Here's how the part is built. I have some questions about the finished solid (model axes, mm). Face numbers are marked on the shaded views. A direction names the side the tool comes from. Round coordinates to 2 decimals unless told otherwise and drop trailing zeros. Loops run counter-clockwise (first coordinate to the right, second up) from the corner with the lowest first, then second, coordinate; pieces in that order, holes last. Notation, with made-up numbers: M -10,-26.5 L 15,-26.5 A17 ccw 15,-13.5 Z; hole C 6,3 d1. An arc over 180 degrees is marked long. Use a Markdown table: item, result.
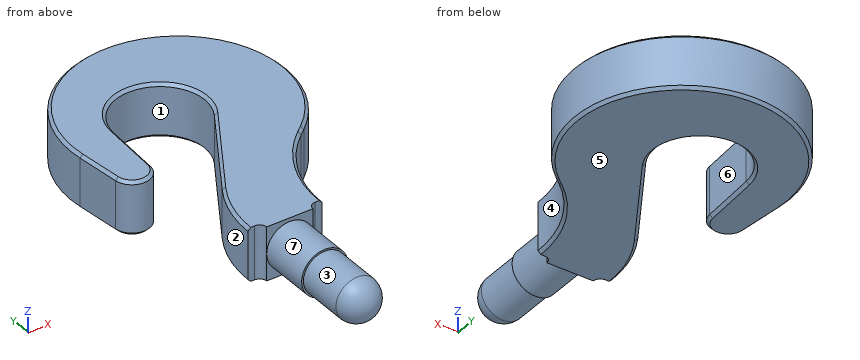
from build123d import *

# Parameters (mm, degrees)
BOSS_EXTRUDE1_DEPTH = 15
CHAMFER1_SIZE       = 0.8
SKETCH2_R           = 6.5
BOSS_EXTRUDE2_DEPTH = 14
SKETCH3_R           = 6
BOSS_EXTRUDE3_DEPTH = 13
DOME1_FACE_RADIUS   = 6
DOME1_HEIGHT        = 5.61


with BuildPart() as part:
    # Sketch1 → Boss-Extrude1 (new body)
    with BuildSketch(Plane.XY):
        with BuildLine():
            Line((5.33, -50.05), (3.429374902, -50.05))
            ThreePointArc((3.429374902, -50.05), (2.032950898, -50.618217894), (1.43, -52))
            Line((1.43, -52), (-11.57, -52))
            ThreePointArc((-11.57, -52), (-12.172950898, -50.618217894), (-13.569374902, -50.05))
            Line((-13.569374902, -50.05), (-15.47, -50.05))
            ThreePointArc((-15.47, -50.05), (-14.21947106, -41.051606397), (-10.562661368, -32.73519774))
            Line((-10.562661368, -32.73519774), (5.571159609, -6.55863722))
            ThreePointArc((5.571159609, -6.55863722), (-1.303288682, 11.918971677), (-17.547628929, 0.747513411))
            Line((-17.547628929, 0.747513411), (-18.508948428, -15.299005365))
            ThreePointArc((-18.508948428, -15.299005365), (-23.375545829, -19.998450876), (-28.469986749, -15.547020759))
            Line((-28.469986749, -15.547020759), (-29.819920496, -3.282124556))
            ThreePointArc((-29.819920496, -3.282124556), (11.287126383, 27.795697113), (19.089371058, -23.142945202))
            Line((19.089371058, -23.142945202), (17.331691836, -24.592760278))
            ThreePointArc((17.331691836, -24.592760278), (8.480844489, -35.977760828), (5.33, -50.05))
        make_face()
    extrude(amount=BOSS_EXTRUDE1_DEPTH)

    # Chamfer1
    chamfer1_edges = [part.edges().sort_by_distance(p)[0] for p in [
        (11.287126383, 27.795697113, 15),
        (-29.144953623, -9.414572658, 15),
        (-14.21947106, -41.051606397, 0),
        (-2.495750879, -19.64691748, 0),
        (-1.303288682, 11.918971677, 0),
        (-18.028288679, -7.275745977, 0),
        (-23.375545829, -19.998450876, 15),
        (-23.375545829, -19.998450876, 0),
        (-29.144953623, -9.414572658, 0),
        (11.287126383, 27.795697113, 0),
        (18.210531447, -23.86785274, 0),
        (8.480844489, -35.977760828, 0),
        (-18.028288679, -7.275745977, 15),
        (-1.303288682, 11.918971677, 15),
        (-2.495750879, -19.64691748, 15),
        (-14.21947106, -41.051606397, 15),
        (8.480844489, -35.977760828, 15),
        (18.210531447, -23.86785274, 15),
    ]]
    chamfer(chamfer1_edges, length=CHAMFER1_SIZE)

    # Sketch2 → Boss-Extrude2 (add)
    with BuildSketch(Plane.XZ.offset(52)):
        with Locations(Location((-5.07, 7.5, 0), (0, 0, 180))):
            Circle(SKETCH2_R)
    extrude(amount=BOSS_EXTRUDE2_DEPTH)

    # Sketch3 → Boss-Extrude3 (add)
    with BuildSketch(Plane.XZ.offset(66)):
        with Locations(Location((-5.07, 7.5, 0), (0, 0, 90))):
            Circle(SKETCH3_R)
    extrude(amount=BOSS_EXTRUDE3_DEPTH)

    # Dome1: a dome of height H over a round flat face of radius A is a cap of a sphere of radius (A * A + H * H) / (2 * H)
    dome1_r = (DOME1_FACE_RADIUS * DOME1_FACE_RADIUS + DOME1_HEIGHT * DOME1_HEIGHT) / (2 * DOME1_HEIGHT)
    dome1_base = Plane((-5.07, -79, 7.5), z_dir=(0, -1, 0))
    with Locations(dome1_base.offset(DOME1_HEIGHT - dome1_r)):
        dome1_ball = Sphere(dome1_r, mode=Mode.PRIVATE)
    add(split(dome1_ball, bisect_by=dome1_base, keep=Keep.TOP, mode=Mode.PRIVATE))


solid = part.part
1. For pin 1 Ø2 at (x, z) = (4.5, 7) entering from -Y; pin 2 Ø1.5 at (x, z) = (14.5, 4) entering from +Y; pin 3 Ø5 at (x, z) = (-19.5, 9) entering from -Y, each with a flat end and sliding along its axis, tell me the tip position at first contact or that it passes through.
Answer sheet:
| item | result |
|---|---|
| pin 1 | y = -50.05 |
| pin 2 | y = 26.66 |
| pin 3 | y = -19.77 |
2. I need wall thicknesses on probe 1 along Y at (x, z) = (-4, 4.75); probe 2 along X at (y, z) = (0, 6.75); probe 3 along X at (y, z) = (4, 5.25). Which ranges of each line are inside material? Lowest first, please. Write a range as from..to.
Answer sheet:
| item | result |
|---|---|
| probe 1 | -83.84..-22.09, 12.45..29.73 |
| probe 2 | -30..-17.59, 7.43..30 |
| probe 3 | -29.73..-16.91, 6.77..29.73 |
3. Imagine slicing it at A-A, the plane z = 9.5. Write out the boundary of the cut face in (x, y).
Answer sheet:
| item | result |
|---|---|
| outline | M -29.82,-3.28 L -28.47,-15.55 A5 ccw -18.51,-15.3 L -17.55,0.75 A12.5 cw long 5.57,-6.56 L -10.56,-32.74 A33 ccw -15.47,-50.05 L -13.57,-50.05 A2 cw -11.57,-52 L -11.25,-52 L -11.25,-66 L -10.73,-66 L -10.73,-79 A5.67 ccw 0.59,-79 L 0.59,-66 L 1.11,-66 L 1.11,-52 L 1.43,-52 A2 cw 3.43,-50.05 L 5.33,-50.05 A33 cw 17.33,-24.59 L 19.09,-23.14 A30 ccw long Z |
4. Which directions (+Z, -Z, +X, -X, +Y, -Y) give clear straight access to the entire face, cutting with the end or side of a thin tool? Please do the marked faces 5, 6 and 7.
Answer sheet:
| item | result |
|---|---|
| face 5 | -Z, +X, -X, +Y, -Y |
| face 6 | +Z, -Z, -Y |
| face 7 | -Y |
5. We'd pull the mould along Y, two halves only. Please class the marked faces 1, 2, 3 and 4: +Y half, -Y half, draft (parallel to the pull), parting line (faces both ways), or undercut.
Answer sheet:
| item | result |
|---|---|
| face 1 | undercut |
| face 2 | undercut |
| face 3 | draft |
| face 4 | -Y half |
6. Imagine slicing it at C-C, the plane z = 3. Write out the boundary of the cut face in (x, y).
Answer sheet:
| item | result |
|---|---|
| outline | M -29.82,-3.28 L -28.47,-15.55 A5 ccw -18.51,-15.3 L -17.55,0.75 A12.5 cw long 5.57,-6.56 L -10.56,-32.74 A33 ccw -15.47,-50.05 L -13.57,-50.05 A2 cw -11.57,-52 L -9.76,-52 L -9.76,-66 L -9.04,-66 L -9.04,-79 A3.99 ccw -1.1,-79 L -1.1,-66 L -0.38,-66 L -0.38,-52 L 1.43,-52 A2 cw 3.43,-50.05 L 5.33,-50.05 A33 cw 17.33,-24.59 L 19.09,-23.14 A30 ccw long Z |
7. Imagine slicing it at B-B, the plane y = -73. Write out the boundary of the cut face in (x, z).
Answer sheet:
| item | result |
|---|---|
| outline | C -5.07,7.5 d12 |
